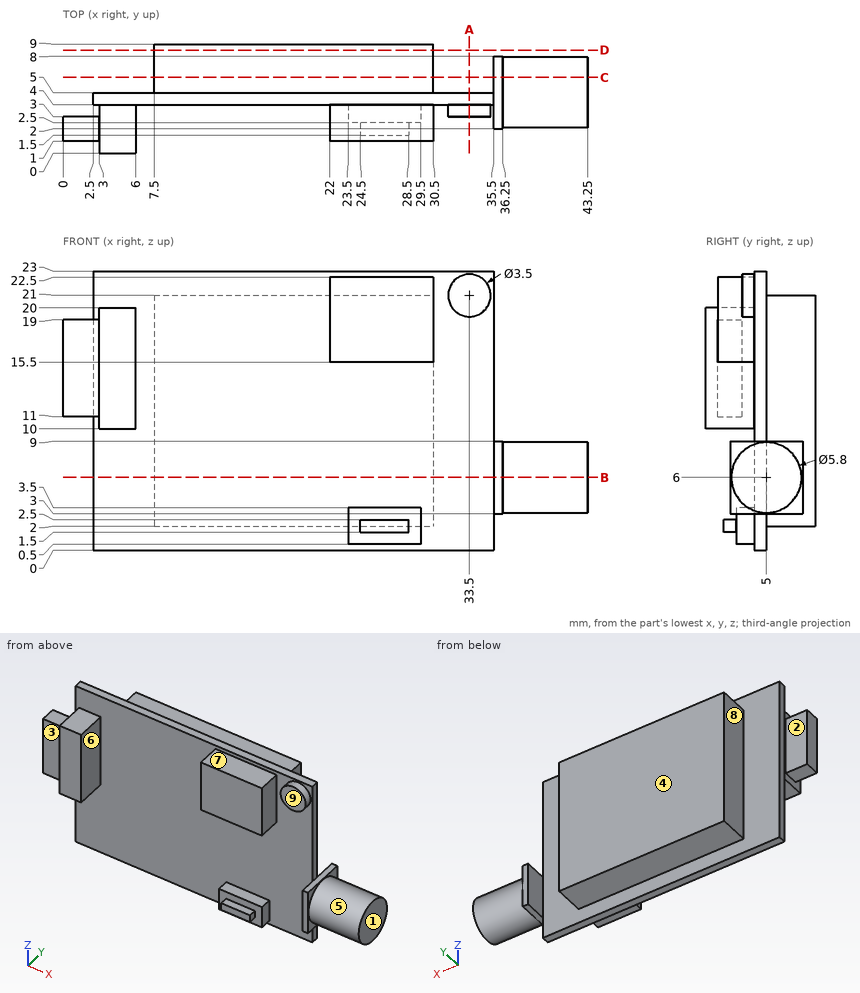
For this review, use the dimensioned drawing (mm, ordinates from the lowest corner) and the shaded views. A direction names the side the tool comes from. Round coordinates to 2 decimals unless told otherwise and drop trailing zeros. Loops run counter-clockwise (first coordinate to the right, second up) from the corner with the lowest first, then second, coordinate; pieces in that order, holes last. Notation, with made-up numbers: (83.5, 39.5) -> (122.5, 39.5) arc R31 ccw to (122.5, 70.5) -> close; hole circle Ø3 at (57.25, 75.5). An arc over 180 degrees is marked (long way). Write item = value, one per line. Start each with the question number.
Item 1: Take a section at B-B on z = 6. Give the boundary of the cut face in (x, y).
Item 2: For the marked faces 5, 6, 7, 8 and 9, list the 3-axis set-ups (+Z, -Z, +X, -X, +Y, -Y) from which the entire face can be reached by the end or side of a thin tool; tool diameter is ignored.
Item 3: Take a section at C-C on y = 6.25. Give the boundary of the cut face in (x, z), plus the area to 3 significant figures.
Item 4: To check wall thickness, follow L1, parallel to X at y = 2.5, z = 5.25; L2, parallel to Z at x = 11, y = 8.75; L3, parallel to Y at x = 29, z = 13.75. State the ranges of each line that lie inside material, in increasing order.
Item 5: Take a section at D-D on y = 8.5. Give the boundary of the cut face in (x, z), plus the area to 3 significant figures.
Item 6: Insertion check: pin 1 (1 mm diameter, centred on y = 4.5, z = 5, fed in from -X); pin 2 (3 mm diameter, centred on x = 21, y = 7.5, fed in from -Z); pin 3 (7.5 mm diameter, centred on x = 26.5, z = 17.5, fed in from -Y). Each pin has a flat end and moves straight along its axis. Give the tip position at first contact, or say it passes through.
Item 7: Take a section at A-A on x = 33.5. Give the boundary of the cut face in (y, z), plus the area to 3 significant figures.
Item 8: Mouldability with a two-part tool opening along Y and no side actions: class the marked faces 1, 2, 3 and 4 as released by +Y, released by -Y, zero draft, split by the parting line, or undercut.
Result:
q1.outline = (2.5, 4) -> (35.5, 4) -> (35.5, 2) -> (36.25, 2) -> (36.25, 2.1) -> (43.25, 2.1) -> (43.25, 7.9) -> (36.25, 7.9) -> (36.25, 8) -> (35.5, 8) -> (35.5, 5) -> (30.5, 5) -> (30.5, 9) -> (7.5, 9) -> (7.5, 5) -> (2.5, 5) -> close
q2.face_5 = +X
q2.face_6 = +Z, -Z, -Y
q2.face_7 = +Z, -X, -Y
q2.face_8 = +Z, -Z, -X, +Y
q2.face_9 = +Z, -Z, +X, -Y
q3.outline = (7.5, 2) -> (30.5, 2) -> (30.5, 21) -> (7.5, 21) -> close; (35.5, 3) -> (36.25, 3) -> (36.25, 3.38) -> (43.25, 3.38) -> (43.25, 8.62) -> (36.25, 8.62) -> (36.25, 9) -> (35.5, 9) -> close
q3.area = 478 mm²
q4.L1 = 35.5 to 43.25
q4.L2 = 2 to 21
q4.L3 = 4 to 9
q5.outline = (7.5, 2) -> (30.5, 2) -> (30.5, 21) -> (7.5, 21) -> close
q5.area = 437 mm²
q6.pin_1 = 2.5
q6.pin_2 = 2
q6.pin_3 = 1
q7.outline = (3, 19.25) -> (4, 19.25) -> (4, 0) -> (5, 0) -> (5, 23) -> (4, 23) -> (4, 22.75) -> (3, 22.75) -> close
q7.area = 26.5 mm²
q8.face_1 = zero draft
q8.face_2 = undercut
q8.face_3 = released by -Y
q8.face_4 = released by +Y
